```python
from build123d import *

# Parameters (mm, degrees)
F0_R     = 9.525
F1_DEPTH = 25.4
F2_W     = 25.4
F2_H     = 76.2
F3_DEPTH = 25.4
F5_DEPTH = 76.201


with BuildPart() as f1:
    # F0 (on Top) → F1 (new body)
    with BuildSketch(Plane.XY):
        Circle(F0_R)
    extrude(amount=F1_DEPTH)

    # F2 (on face) → F3 (join)
    with BuildSketch(Plane(origin=(0, 0, 0), x_dir=(1, 0, 0), z_dir=(0, 0, -1))):
        Rectangle(F2_W, F2_H)
    extrude(amount=F3_DEPTH)

    # F4 (on face) → F5 (cut, through all)
    with BuildSketch(Plane.XZ.offset(38.1)):
        Polygon((12.7, -25.4), (12.7, 0), (-12.7, -25.4), align=None)
    extrude(amount=-F5_DEPTH, mode=Mode.SUBTRACT)


solid = f1.part
```
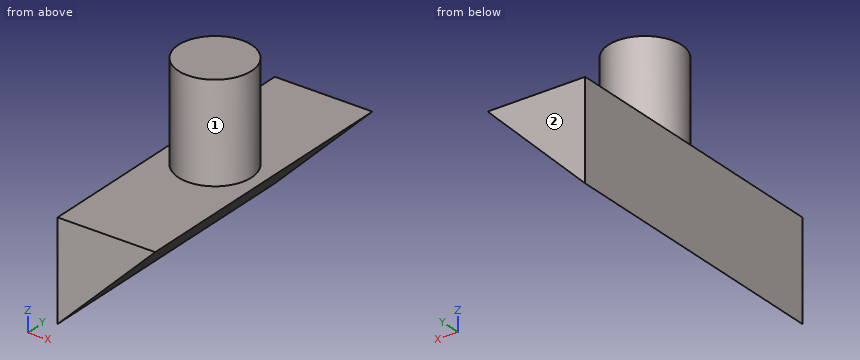
The listing builds one solid part. Answer for the finished solid, in the listing's coordinates (mm). Face numbers are marked on the shaded views. A direction names the side the tool comes from. Round coordinates to 2 decimals unless told otherwise and drop trailing zeros. Write each loop counter-clockwise with the first axis right and the second up, starting at its lowest first coordinate (ties: lowest second). Pieces come first, ordered by that corner, then holes. Notation, with made-up numbers: (46, 79.25) -> (68, 79.25) arc R25 cw to (68, 106.25) -> close; hole circle Ø5 at (29, 86.5). An arc over 180 degrees is marked (long way). Write item = value, one per line.
1) Section A-A on y = 0 is taken. Write down the section's boundary in (x, z) (3 decimals).
Check values:
outline = (-12.7, -25.4) -> (12.7, 0) -> (9.525, 0) -> (9.525, 25.4) -> (-9.525, 25.4) -> (-9.525, 0) -> (-12.7, 0) -> close
2) Section C-C on z = -11.5 is taken. Write down the section's boundary in (x, y).
Check values:
outline = (-12.7, -38.1) -> (1.2, -38.1) -> (1.2, 38.1) -> (-12.7, 38.1) -> close
3) Given pin 1 (5 mm diameter, centred on x = 1.5, y = 13, fed in from +Z); pin 2 (4 mm diameter, centred on x = 9, z = 4.5, fed in from -Y); pin 3 (1 mm diameter, centred on x = -0.5, y = 18, fed in from -Z), each flat-ended and moving along its own axis, determine where each tip first touches the part or whether it passes through.
Check values:
pin_1 = 0
pin_2 = -6.46
pin_3 = -13.7
4) Section D-D on x = -8.5 is taken. Write down the section's boundary in (y, z), plus the area to 3 significant figures.
Check values:
outline = (-38.1, -21.2) -> (38.1, -21.2) -> (38.1, 0) -> (4.3, 0) -> (4.3, 25.4) -> (-4.3, 25.4) -> (-4.3, 0) -> (-38.1, 0) -> close
area = 1,830 mm²
5) Which of the six approach directions +Z, -Z, +X, -X, +Y, -Y give full straight-line access (tool end or side, diameter ignored) to the marked faces 1 and 2?
Check values:
face_1 = +Z
face_2 = +Z, -Z, +X, -X, +Y
6) Section B-B on x = 0 is taken. Write down the section's boundary in (y, z) (3 decimals).
Check values:
outline = (-38.1, -12.7) -> (38.1, -12.7) -> (38.1, 0) -> (9.525, 0) -> (9.525, 25.4) -> (-9.525, 25.4) -> (-9.525, 0) -> (-38.1, 0) -> close
7) Straight lines are drawn through the part: line 1 along X through (y, z) = (26, -21.5); line 2 along Z through (x, y) = (6.25, 12); line 3 along X through (y, z) = (13.5, -8). For each, find the intervals that lie inside material, in ascending order. Write a range as [from, to].
Check values:
line_1 = [-12.7, -8.8]
line_2 = [-6.45, 0]
line_3 = [-12.7, 4.7]
